Here's how the part is built. I have some questions about the finished solid (model axes, mm). Coordinates: 2 decimals unless noted, no trailing zeros. Loops run counter-clockwise (first coordinate to the right, second up) from the corner with the lowest first, then second, coordinate; pieces in that order, holes last. Notation, with made-up numbers: M 57,10.25 L 67,10.25 A9 ccw 67,21.25 Z; hole C -13.75,83 d3. An arc over 180 degrees is marked long. Use one line per item in the form item = value. Start each with the question number.
(1) Will these pins go through, and if not, where does the flat tip stop? P1, Ø12, axis at x = 3, z = 724, coming from the -Y side; P2, Ø1, axis at x = -0.5, z = 1241.5, coming from the +Y side; P3, Ø4, axis at x = 4.5, z = 850, coming from the -Y side; P4, Ø6, axis at y = -1.5, z = 469.5, coming from the -X side.
(2) Imagine slicing it at A-A, the plane z = 1107.5. Please give me the cut outline in (x, y), and give its area (3 significant figures).
(3) Imagine slicing it at B-B, the plane y = 2.75. Please give me the cut outline in (x, z), and give its area (3 significant figures).
(4) Please list where these lines run through material, in increasing order: L1, parallel to Y at x = 17, z = 1171; L2, parallel to X at y = -11.5, z = 590.5; L3, parallel to Y at x = 2, z = 1158.
```python
from build123d import *

# Parameters (mm, degrees)
SKETCH2_W           = 40
SKETCH2_H           = 30
BOSS_EXTRUDE2_DEPTH = 1500
SKETCH3_W           = 15
SKETCH3_H           = 5
SKETCH3_W_2         = 5
SKETCH3_H_2         = 15
CUT_EXTRUDE1_DEPTH  = 1500


with BuildPart() as part:
    # Sketch2 → Boss-Extrude2 (new body)
    with BuildSketch(Plane.XY):
        Rectangle(SKETCH2_W, SKETCH2_H)
    extrude(amount=BOSS_EXTRUDE2_DEPTH)

    # Sketch3 → Cut-Extrude1 (cut)
    with BuildSketch(Plane.XY.offset(1500)):
        with Locations((0, 12.5)):
            Rectangle(SKETCH3_W, SKETCH3_H)
        with Locations((17.5, 0)):
            Rectangle(SKETCH3_W_2, SKETCH3_H_2)
        with Locations((0, -12.5)):
            Rectangle(SKETCH3_W, SKETCH3_H)
        with Locations((-17.5, 0)):
            Rectangle(SKETCH3_W_2, SKETCH3_H_2)
    extrude(amount=-CUT_EXTRUDE1_DEPTH, mode=Mode.SUBTRACT)


solid = part.part
```
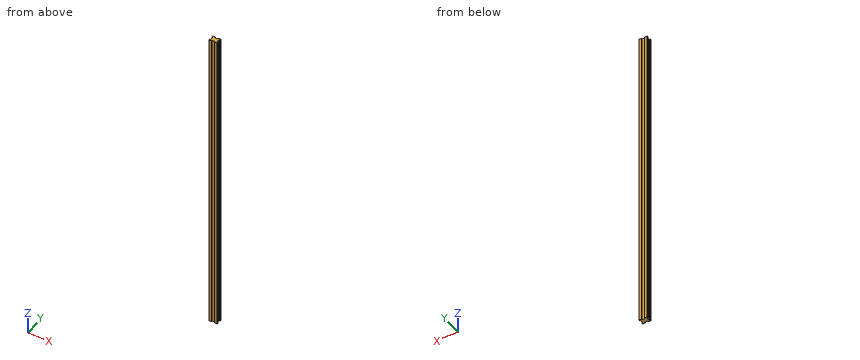
Answer:
q1.P1 = -15
q1.P2 = 10
q1.P3 = -10
q1.P4 = -15
q2.outline = M -20,-15 L -7.5,-15 L -7.5,-10 L 7.5,-10 L 7.5,-15 L 20,-15 L 20,-7.5 L 15,-7.5 L 15,7.5 L 20,7.5 L 20,15 L 7.5,15 L 7.5,10 L -7.5,10 L -7.5,15 L -20,15 L -20,7.5 L -15,7.5 L -15,-7.5 L -20,-7.5 Z
q2.area = 900 mm²
q3.outline = M -15,0 L 15,0 L 15,1500 L -15,1500 Z
q3.area = 45,000 mm²
q4.L1 = -15 to -7.5, 7.5 to 15
q4.L2 = -20 to -7.5, 7.5 to 20
q4.L3 = -10 to 10
